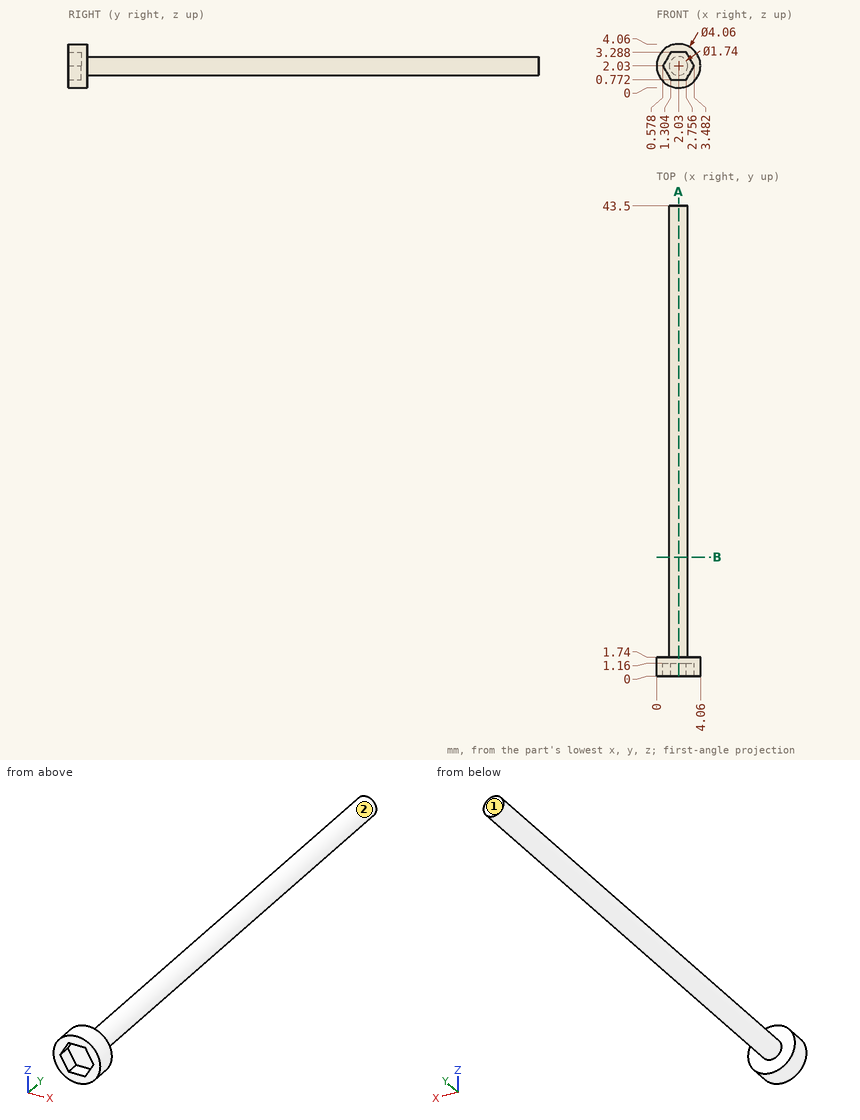
Can you work these out from the drawing? Everything is in mm from the part's minimum corner. A direction names the side the tool comes from. Round coordinates to 2 decimals unless told otherwise and drop trailing zeros. Loops run counter-clockwise (first coordinate to the right, second up) from the corner with the lowest first, then second, coordinate; pieces in that order, holes last. Notation, with made-up numbers: M -27,-10 L 30,-10 A22 ccw 30,16 Z; hole C 28.25,16.5 d1. An arc over 180 degrees is marked long. Answer in a Markdown table with one row per item.
1. If we section it at A-A, the plane x = 2.03: Please give me the cut outline in (y, z).
Established:
| item | result |
|---|---|
| outline | M 0,0 L 1.74,0 L 1.74,1.16 L 43.5,1.16 L 43.5,2.9 L 1.74,2.9 L 1.74,4.06 L 0,4.06 L 0,3.29 L 1.16,3.29 L 1.16,0.77 L 0,0.77 Z |
2. On a 3-axis mill with a long thin cutter (end or side, diameter ignored), from which of +Z, -Z, +X, -X, +Y, -Y can I reach the whole of each face in a straight line? I mean the marked faces 1 and 2. Say none if no direction works.
Established:
| item | result |
|---|---|
| face 1 | +Z, -Z, +X, -X, +Y |
| face 2 | +Y |
3. Please list where these lines run through material, in increasing order: line 1 (Y direction, x = 1.1, z = 1.25); line 2 (Y direction, x = 0.55, z = 2.4); line 3 (Z direction, x = 2.5, y = 35). Write a range as from..to.
Established:
| item | result |
|---|---|
| line 1 | 1.16..1.74 |
| line 2 | 0..1.74 |
| line 3 | 1.3..2.76 |
4. If we section it at B-B, the plane y = 11: Please give me the cut outline in (x, z).
Established:
| item | result |
|---|---|
| outline | C 2.03,2.03 d1.74 |
